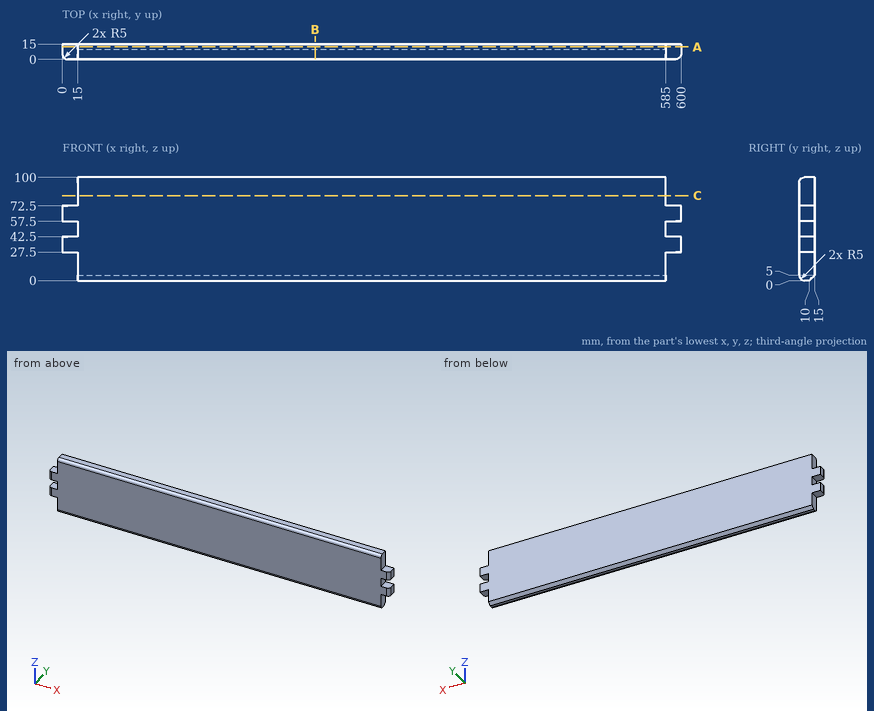
Job drawing, mm, ordinate dimensions from the low corner. One solid piece. Coordinates: 2 decimals unless noted, no trailing zeros. Loops run counter-clockwise (first coordinate to the right, second up) from the corner with the lowest first, then second, coordinate; pieces in that order, holes last. Notation, with made-up numbers: (54.25, -4) - (92.25, -4) arc R13 ccw to (92.25, 18) - close; hole circle Ø8 at (29.25, -6). An arc over 180 degrees is marked (long way). Write item = value, one per line. Start each with the question number.
Q1. Drill centre lines: L1, parallel to X at y = 14.25, z = 78; L2, parallel to Z at x = 459.5, y = 11; L3, parallel to Z at x = 278.5, y = 11.75. Where is each one in solid material? Low to high.
Q2. Cut at B-B, the plane x = 245. List the corners of the cut face in (y, z), then the cut area to 3 significant figures.
Q3. Cut at C-C, the plane z = 82.5. List the corners of the cut face in (x, y).
Q4. Cut at A-A, the plane y = 12.25. List the corners of the cut face in (x, z), then the cut area to 3 significant figures.
Q5. Flat gauge pins, fed straight in: pin 1 Ø5 at (x, y) = (158.5, 5) entering from -Z; pin 2 Ø7.5 at (x, y) = (11, 6.5) entering from -Z; pin 3 Ø1 at (x, y) = (458.5, 3) entering from +Z; pin 4 Ø4.5 at (y, z) = (4, 49.5) entering from -X. Where does each tip first touch, or does it go through?
Computed:
q1.L1 = 15 to 585
q1.L2 = 1 to 100
q1.L3 = 1.75 to 100
q2.outline = (0, 5) arc R5 ccw to (5, 0) - (10, 0) - (15, 5) - (15, 100) - (5, 100) arc R5 ccw to (0, 95) - close
q2.area = 1,480 mm²
q3.outline = (15, 0) - (585, 0) - (585, 15) - (15, 15) - close
q4.outline = (0, 27.5) - (15, 27.5) - (15, 2.25) - (585, 2.25) - (585, 27.5) - (600, 27.5) - (600, 42.5) - (585, 42.5) - (585, 57.5) - (600, 57.5) - (600, 72.5) - (585, 72.5) - (585, 100) - (15, 100) - (15, 72.5) - (0, 72.5) - (0, 57.5) - (15, 57.5) - (15, 42.5) - (0, 42.5) - close
q4.area = 56,600 mm²
q5.pin_1 = 0
q5.pin_2 = 27.5
q5.pin_3 = 99.77
q5.pin_4 = 15
